The listing builds one solid part. Answer for the finished solid, in the listing's coordinates (mm). Face numbers are marked on the shaded views. A direction names the side the tool comes from. Round coordinates to 2 decimals unless told otherwise and drop trailing zeros. Write each loop counter-clockwise with the first axis right and the second up, starting at its lowest first coordinate (ties: lowest second). Pieces come first, ordered by that corner, then holes.
Item 1: Find section A-A on z = -5. Give the vertices of the cut face in (x, y).
Item 2: Find section B-B on y = -33.75. Give the vertices of the cut face in (x, z).
Item 3: A tool of negligible diameter and unlimited length cuts with its end or side. For the marked faces 4 and 5, from which of +Z, -Z, +X, -X, +Y, -Y can it reach the whole face along a straight path? Write none if from no direction.
Item 4: Each of these flat-tipped pins is pushed along its axis until it touches: pin 1 (5 mm diameter, centred on x = -51.5, z = -7, fed in from +Y); pin 2 (3 mm diameter, centred on x = -47, z = -6, fed in from +Y); pin 3 (1.2 mm diameter, centred on x = -53.5, z = -5, fed in from +Y). Where does it stop, or does it pass through?
Item 5: Find the intervals of material crossed by probe 1 along X at (y, z) = (-34.5, -4.5); probe 2 along X at (y, z) = (-33.5, -1.5); probe 3 along Y at (x, z) = (-52.5, -4.5), in increasing order.
Item 6: Find section C-C on x = -47.75. Give the vertices of the cut face in (y, z).
Item 7: For a pull along X with two mould halves and no side action, classify the marked faces 1, 2 and 3 as +X half, -X half, draft (parallel to the pull), parting line (faces both ways), or undercut.
```python
from build123d import *

# Parameters (mm, degrees)
SKETCH1_W                 = 230
SKETCH1_H                 = 6
BOSS_EXTRUDE1_DEPTH       = 9
BOSS_EXTRUDE2_DEPTH       = 9
LPATTERN1_COUNT           = 41
LPATTERN1_PITCH           = 5.5
SKETCH2_W                 = 15
SKETCH2_H                 = 20
BOSS_EXTRUDE3_DEPTH       = 5
FILLET1_R                 = 10
FILLET2_R                 = 3
SKETCH3_W                 = 13
SKETCH3_H                 = 8
BOSS_EXTRUDE4_DEPTH       = 5
SKETCH4_W                 = 3
SKETCH4_H                 = 8
BOSS_EXTRUDE5_DEPTH       = 5
FILLET3_R                 = 0.4
F_3_0MM_DOWEL_HOLE1_D     = 2.7
F_3_0MM_DOWEL_HOLE1_DEPTH = 7
F_3_0MM_DOWEL_HOLE1_TIP   = 0.811161836
SKETCH6_W                 = 22.006931309
SKETCH6_H                 = 16.378230192
SKETCH6_W_2               = 21.806931309
SKETCH6_H_2               = 16.178230192
CUT_EXTRUDE1_DEPTH        = 180.611613715


with BuildPart() as part:
    # Sketch1 → Boss-Extrude1 (new body)
    with BuildSketch(Plane.XY):
        with Locations((54.307342656, -37.82930415)):
            Rectangle(SKETCH1_W, SKETCH1_H)
    extrude(amount=-BOSS_EXTRUDE1_DEPTH)

    # Sketch1<3> → Boss-Extrude2 (add)
    with BuildSketch(Plane.XY):
        with BuildLine():
            ThreePointArc((-56.340727793, -31.82930415), (-57.041926016, -33.262238075), (-57.340727793, -34.82930415))
            Line((-57.340727793, -34.82930415), (-54.340727793, -34.82930415))
            ThreePointArc((-54.340727793, -34.82930415), (-54.63952957, -33.262238075), (-55.340727793, -31.82930415))
            Line((-55.340727793, -31.82930415), (-56.340727793, -31.82930415))
        make_face()
    boss_extrude2 = extrude(amount=-BOSS_EXTRUDE2_DEPTH)

    # LPattern1: Boss-Extrude2 ×41
    with Locations(*[(i * LPATTERN1_PITCH, 0, 0) for i in range(1, LPATTERN1_COUNT)]):
        add(boss_extrude2)

    # Sketch2 → Boss-Extrude3 (add)
    with BuildSketch(Plane.XZ.offset(40.82930415)):
        with Locations((-68.192657344, -4.5)):
            Rectangle(SKETCH2_W, SKETCH2_H)
    extrude(amount=-BOSS_EXTRUDE3_DEPTH)

    # Fillet1
    # the kernel refuses this fillet: 10 mm, written as the material it adds along each edge
    with BuildSketch(Plane(origin=(-60.692657344, -35.82930415, 0), x_dir=(0, 1, 0), z_dir=(0, 0, -1))) as fillet1_piece_1:
        with BuildLine():
            CenterArc((10, -4.358898944), FILLET1_R, 154.158067237, 25.841932763)
            Line((0, -4.358898944), (0, 0))
            Line((0, 0), (1, 0))
        make_face()
    extrude(amount=9)

    # Fillet2
    fillet2_edges = [part.edges().sort_by_distance(p)[0] for p in [
        (-60.692657344, -38.32930415, 5.5),
        (-60.692657344, -38.32930415, -14.5),
        (-75.692657344, -38.32930415, -14.5),
        (-75.692657344, -38.32930415, 5.5),
    ]]
    fillet(fillet2_edges, radius=FILLET2_R)

    # Sketch3 → Boss-Extrude4 (add)
    with BuildSketch(Plane(origin=(169.307342656, 0, 0), x_dir=(0, 0, -1), z_dir=(1, 0, 0))):
        with Locations((4.5, -36.82930415)):
            Rectangle(SKETCH3_W, SKETCH3_H)
    extrude(amount=BOSS_EXTRUDE4_DEPTH)

    # Sketch4 → Boss-Extrude5 (add)
    with BuildSketch(Plane.XY.offset(2)):
        with Locations((170.807342656, -36.82930415)):
            Rectangle(SKETCH4_W, SKETCH4_H)
    extrude(amount=BOSS_EXTRUDE5_DEPTH)

    # Fillet3
    fillet3_edges = [part.edges().sort_by_distance(p)[0] for p in [
        (54.307342656, -40.82930415, -9),
        (-60.692657344, -40.82930415, 1.25),
        (-68.192657344, -40.82930415, -14.5),
        (-68.192657344, -40.82930415, 5.5),
        (-75.692657344, -40.82930415, -4.5),
        (-60.692657344, -40.82930415, -10.25),
        (-61.571337, -40.82930415, 4.621320344),
        (-74.813977688, -40.82930415, 4.621320344),
        (-74.813977688, -40.82930415, -13.621320344),
        (-61.571337, -40.82930415, -13.621320344),
        (173.307342656, -32.82930415, 2),
        (169.307342656, -40.82930415, 3.5),
        (169.307342656, -40.82930415, -10),
        (173.307342656, -40.82930415, 2),
        (171.807342656, -40.82930415, -11),
        (169.307342656, -32.82930415, -2),
        (171.807342656, -32.82930415, -11),
        (174.307342656, -36.82930415, 2),
        (174.307342656, -40.82930415, -4.5),
        (174.307342656, -36.82930415, -11),
        (174.307342656, -32.82930415, -4.5),
        (172.307342656, -36.82930415, 2),
        (172.307342656, -40.82930415, 4.5),
        (172.307342656, -32.82930415, 4.5),
        (169.307342656, -36.82930415, 7),
        (170.807342656, -40.82930415, 7),
        (172.307342656, -36.82930415, 7),
        (170.807342656, -32.82930415, 7),
        (54.307342656, -40.82930415, 0),
    ]]
    fillet(fillet3_edges, radius=FILLET3_R)

    # Ø3.0mm Dowel Hole1
    with Locations(Plane(origin=(-65.692657344, -40.82930415, 1.5), x_dir=(0, 0, -1), z_dir=(0, -1, 0))):
        with Locations((0, 0), (12, 0), (5.991996797, -6)):
            Hole(F_3_0MM_DOWEL_HOLE1_D / 2, depth=F_3_0MM_DOWEL_HOLE1_DEPTH)
            with Locations((0, 0, -(F_3_0MM_DOWEL_HOLE1_DEPTH + F_3_0MM_DOWEL_HOLE1_TIP / 2))):  # 118° drill point
                Cone(0, F_3_0MM_DOWEL_HOLE1_D / 2, F_3_0MM_DOWEL_HOLE1_TIP, mode=Mode.SUBTRACT)

    # Sketch6 → Cut-Extrude1 (cut, through all)
    with BuildSketch(Plane.XY):
        with Locations((-47.571737998, -32.740189054)):
            Rectangle(SKETCH6_W, SKETCH6_H)
        with Locations((-47.571737998, -32.740189054)):
            Rectangle(SKETCH6_W_2, SKETCH6_H_2, mode=Mode.SUBTRACT)
    extrude(amount=-CUT_EXTRUDE1_DEPTH, mode=Mode.SUBTRACT)


with BuildPart() as cut_extrude1_piece_1:
    # of the separate pieces the step leaves, piece 1, a body of its own (cut_extrude1_pieces)
    add(part.part.solids().sort_by_distance((-36.568272343, -40.82930415, -8.6))[0])


with BuildPart() as cut_extrude1_piece_2:
    # of the separate pieces the step leaves, piece 2, a body of its own (cut_extrude1_pieces)
    add(part.part.solids().sort_by_distance((-58.575203652, -40.82930415, -0.4))[0])


with BuildPart() as cut_extrude1_piece_3:
    # of the separate pieces the step leaves, piece 3, a body of its own (cut_extrude1_pieces)
    add(part.part.solids().sort_by_distance((-58.475203652, -40.82930415, -8.6))[0])


solid = cut_extrude1_piece_3.part
```
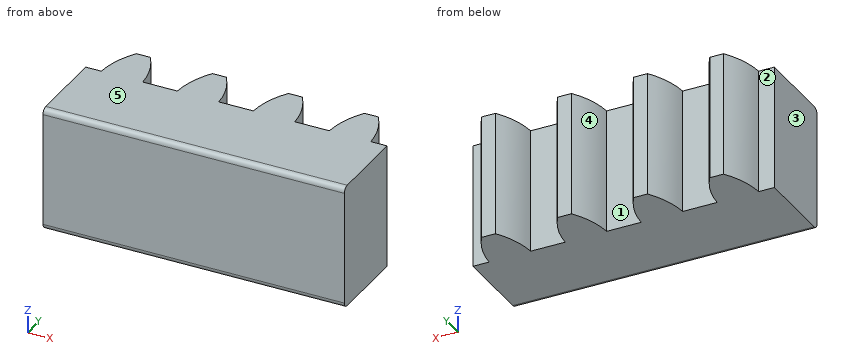
Check values:
1. outline: (-58.48, -40.83) - (-36.67, -40.83) - (-36.67, -34.83) - (-37.84, -34.83) arc R6 ccw to (-38.84, -31.83) - (-39.84, -31.83) arc R6 ccw to (-40.84, -34.83) - (-43.34, -34.83) arc R6 ccw to (-44.34, -31.83) - (-45.34, -31.83) arc R6 ccw to (-46.34, -34.83) - (-48.84, -34.83) arc R6 ccw to (-49.84, -31.83) - (-50.84, -31.83) arc R6 ccw to (-51.84, -34.83) - (-54.34, -34.83) arc R6 ccw to (-55.34, -31.83) - (-56.34, -31.83) arc R6 ccw to (-57.34, -34.83) - (-58.48, -34.83) - close
2. outline: (-57.18, -9) - (-54.5, -9) - (-54.5, 0) - (-57.18, 0) - close; (-51.68, -9) - (-49, -9) - (-49, 0) - (-51.68, 0) - close; (-46.18, -9) - (-43.5, -9) - (-43.5, 0) - (-46.18, 0) - close; (-40.68, -9) - (-38, -9) - (-38, 0) - (-40.68, 0) - close
3. face 4: +Z, -Z, +Y
3. face 5: +Z, +X, -X, +Y, -Y
4. pin 1: stops at y = -31.83
4. pin 2: stops at y = -32.08
4. pin 3: stops at y = -34.83
5. probe 1: x = -57.31 to -54.37, -51.81 to -48.87, -46.31 to -43.37, -40.81 to -37.87
5. probe 2: x = -57.12 to -54.57, -51.62 to -49.07, -46.12 to -43.57, -40.62 to -38.07
5. probe 3: y = -40.83 to -34.83
6. outline: (-40.83, -8.6) arc R0.4 ccw to (-40.43, -9) - (-34.83, -9) - (-34.83, 0) - (-40.43, 0) arc R0.4 ccw to (-40.83, -0.4) - close
7. face 1: undercut
7. face 2: draft
7. face 3: -X half
